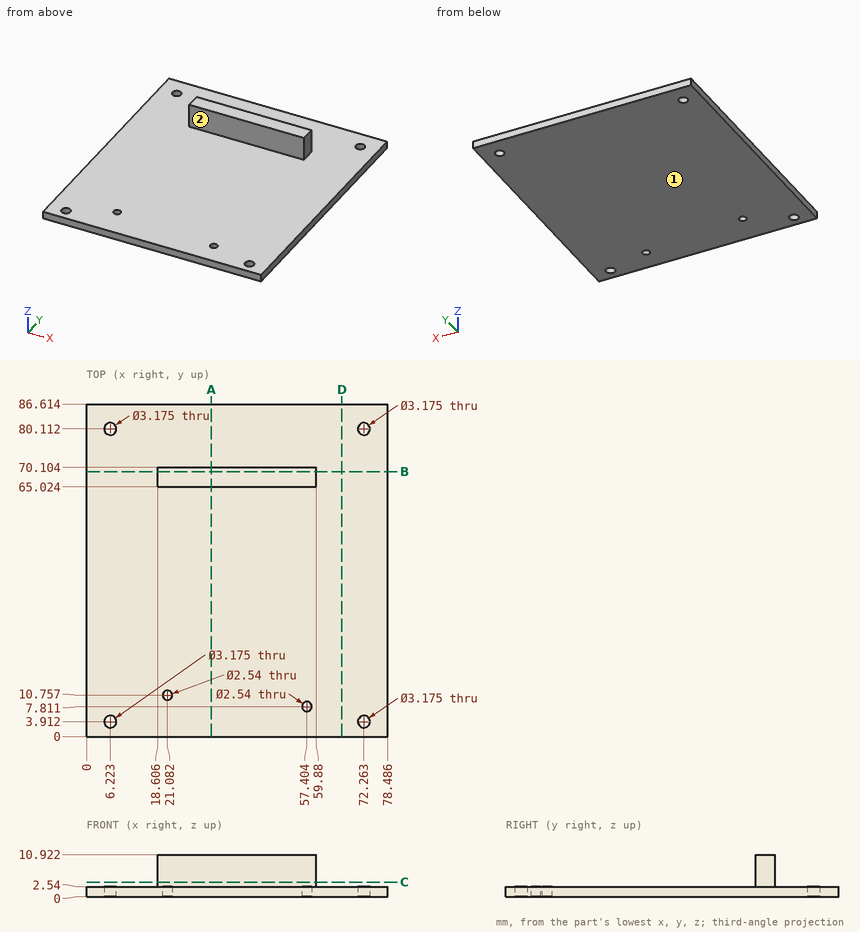
Geometry check sheet. Reference: drawing and pictorial views, mm from the part's lowest x, y, z. A direction names the side the tool comes from. Give positions to 0.01 mm unless a question says otherwise; leave off trailing zeros. Order: outer loops, then holes, each group sorted by start corner. A loop starts at its lowest first (then second) coordinate and runs counter-clockwise, first axis right, second up. Notation, with made-up numbers: M 24,63.5 L 82,63.5 A25 ccw 82,84.5 Z; hole C 8,2.5 d5. An arc over 180 degrees is marked long. Answer in a Markdown table with one row per item.
1) Cross-section at D-D, the plane x = 66.5. Enter the section's corners in (y, z) (1 decimal), plus the area to 3 significant figures.
Filled sheet:
| item | result |
|---|---|
| outline | M 0,0 L 86.6,0 L 86.6,2.5 L 0,2.5 Z |
| area | 220 mm2 |
2) Gauge pin test, flat ends, axial feed: P1, Ø2, axis at x = 64, y = 28.5, coming from the +Z side; P2, Ø1.5, axis at x = 23.5, y = 30.5, coming from the -Z side; P3, Ø4, axis at x = 48, z = 7, coming from the -Y side; P4, Ø4, axis at x = 46, z = 7, coming from the +Y side. Record the tip position at first contact, or that the pin passes through.
Filled sheet:
| item | result |
|---|---|
| P1 | stops at z = 2.54 |
| P2 | stops at z = 0 |
| P3 | stops at y = 65.02 |
| P4 | stops at y = 70.1 |
3) Cross-section at C-C, the plane z = 3.75. Enter the section's corners in (x, y) (1 decimal), plus the area to 3 significant figures.
Filled sheet:
| item | result |
|---|---|
| outline | M 18.6,65 L 59.9,65 L 59.9,70.1 L 18.6,70.1 Z |
| area | 210 mm2 |
4) Cross-section at B-B, the plane y = 69. Enter the section's corners in (x, z) (1 decimal).
Filled sheet:
| item | result |
|---|---|
| outline | M 0,0 L 78.5,0 L 78.5,2.5 L 59.9,2.5 L 59.9,10.9 L 18.6,10.9 L 18.6,2.5 L 0,2.5 Z |
5) Thickness scan on L1, parallel to X at y = 68, z = 7.5 (1 decimal); L2, parallel to Z at x = 3, y = 64.5; L3, parallel to Y at x = 51, z = 9.75 (1 decimal). Record the ranges inside material, lowest first. Write a range as [from, to].
Filled sheet:
| item | result |
|---|---|
| L1 | x = [18.6, 59.9] |
| L2 | z = [0, 2.54] |
| L3 | y = [65, 70.1] |
6) Cross-section at A-A, the plane x = 32.5. Enter the section's corners in (y, z) (1 decimal).
Filled sheet:
| item | result |
|---|---|
| outline | M 0,0 L 86.6,0 L 86.6,2.5 L 70.1,2.5 L 70.1,10.9 L 65,10.9 L 65,2.5 L 0,2.5 Z |
7) Access from +Z, -Z, +X, -X, +Y, -Y to the whole of each face (thin tool, end or side, straight path). Record for the marked faces 1 and 2.
Filled sheet:
| item | result |
|---|---|
| face 1 | -Z, +X, -X, +Y, -Y |
| face 2 | +Z, +X, -X, -Y |
